Study the drawing (mm; zero at the part's minimum x, y, z) and answer. A direction names the side the tool comes from. Coordinates: 2 decimals unless noted, no trailing zeros. Loops run counter-clockwise (first coordinate to the right, second up) from the corner with the lowest first, then second, coordinate; pieces in that order, holes last. Notation, with made-up numbers: (67, 88) -> (92, 88) arc R29 ccw to (92, 113) -> close; hole circle Ø5 at (29, -11). An arc over 180 degrees is marked (long way). One line per question, with ' | ' between items. Start each with the question number.
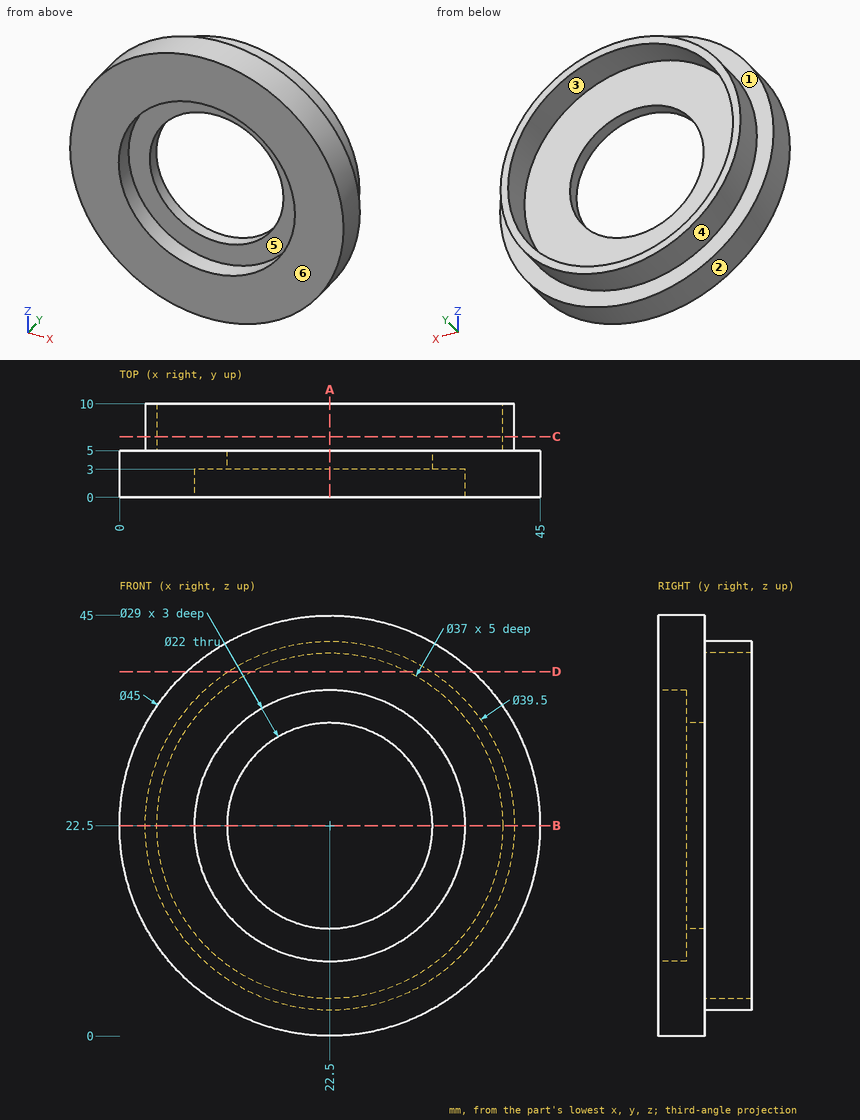
(1) Determine the mould class of the marked faces 3, 4, 5 and 6 for opening direction Z: +Z half, -Z half, draft (parallel to the pull), parting line (faces both ways), or undercut.
(2) Each of these flat-tipped pins is pushed along its axis until it touches: pin 1 Ø5 at (x, y) = (30.5, 4) entering from +Z; pin 2 Ø1.5 at (y, z) = (3, 30.5) entering from +X; pin 3 Ø1 at (x, y) = (19.5, 2.5) entering from +Z; pin 4 Ø14.5 at (x, z) = (28.5, 28) entering from -Y. Where does it stop, or does it pass through?
(3) Section D-D on z = 39 is taken. Write down the section's boundary in (x, y), plus the area to 3 significant figures.
(4) Section C-C on y = 6.5 is taken. Write down the section's boundary in (x, z).
(5) A tool of negligible diameter and unlimited length cuts with its end or side. For the marked faces 1 and 2, from which of +Z, -Z, +X, -X, +Y, -Y can it reach the whole face along a straight path? Write none if from no direction.
(6) Section B-B on z = 22.5 is taken. Write down the section's boundary in (x, y).
(7) Section A-A on x = 22.5 is taken. Write down the section's boundary in (y, z).
(8) Find the intervals of material crossed by probe 1 along Z at (x, y) = (22.5, 7.1); probe 2 along Z at (x, y) = (22.5, 4.3), in increasing order. Write a range as from..to.
Working result:
1) face 3: undercut | face 4: parting line | face 5: undercut | face 6: draft
2) pin 1: stops at z = 44.32 | pin 2: stops at x = 43.8 | pin 3: stops at z = 44.86 | pin 4: stops at y = 0
3) outline: (7.2, 0) -> (37.8, 0) -> (37.8, 5) -> (33.35, 5) -> (33.35, 10) -> (30.87, 10) -> (30.87, 5) -> (14.13, 5) -> (14.13, 10) -> (11.65, 10) -> (11.65, 5) -> (7.2, 5) -> close | area: 178 mm2
4) outline: circle Ø39.5 at (22.5, 22.5); hole circle Ø37 at (22.5, 22.5)
5) face 1: +Y | face 2: +Y, -Y
6) outline: (0, 0) -> (8, 0) -> (8, 3) -> (11.5, 3) -> (11.5, 5) -> (4, 5) -> (4, 10) -> (2.75, 10) -> (2.75, 5) -> (0, 5) -> close; (33.5, 3) -> (37, 3) -> (37, 0) -> (45, 0) -> (45, 5) -> (42.25, 5) -> (42.25, 10) -> (41, 10) -> (41, 5) -> (33.5, 5) -> close
7) outline: (0, 0) -> (5, 0) -> (5, 2.75) -> (10, 2.75) -> (10, 4) -> (5, 4) -> (5, 11.5) -> (3, 11.5) -> (3, 8) -> (0, 8) -> close; (0, 37) -> (3, 37) -> (3, 33.5) -> (5, 33.5) -> (5, 41) -> (10, 41) -> (10, 42.25) -> (5, 42.25) -> (5, 45) -> (0, 45) -> close
8) probe 1: z = 2.75..4, 41..42.25 | probe 2: z = 0..11.5, 33.5..45
